Could you check a few things on this model? Use its own coordinates, in mm. A direction names the side the tool comes from. Round coordinates to 2 decimals unless told otherwise and drop trailing zeros. Write each loop counter-clockwise with the first axis right and the second up, starting at its lowest first coordinate (ties: lowest second). Pieces come first, ordered by that corner, then holes. Notation, with made-up numbers: M 14,60.5 L 52,60.5 A29 ccw 52,83.5 Z; hole C 46,-30.75 d11. An arc over 180 degrees is marked long. One line per item, written item: value. Start each with the question number.
(1) I want a section at A-A on y = -12. Please give me the cut outline in (x, z).
(2) Which directions (+Z, -Z, +X, -X, +Y, -Y) give clear straight access to the entire face, cutting with the end or side of a thin tool? Please do faces 1 (the face through (9.13, 17.26, -17.32)), 2 (the face through (75, -10, -68)), 3 (the face through (51, -10, -140)).
(3) Thinking about a two-plate mould opening in Y: for faces 4 (the face through (21, 75, -136)), 5 (the face through (29.84, 82.5, -120.4)), 6 (the face through (82.13, -9.86, -123.07)), which applies, released by +Y, released by -Y, zero draft, split by the parting line, or undercut?
(4) I'm going to push flat-ended pins straight in: pin 1 Ø12 at (x, y) = (23, 56) entering from -Z; pin 2 Ø7.5 at (x, z) = (6.5, -8) entering from +Y; pin 3 Ø16 at (x, y) = (49.5, -6.5) entering from -Z; pin 4 Ø13.5 at (x, z) = (85, -130) entering from -Y. Where does each tip first touch, or does it pass through?
(5) I want a section at D-D on x = 7.5. Please give me the cut outline in (y, z).
(6) I want a section at C-C on z = -125.5. Please give me the cut outline in (x, y), and give its area (3 significant figures).
(7) If I drill on L1, parallel to X at y = 3.5, z = -9.5; L2, parallel to X at y = -15.5, z = -130; L3, parallel to Z at x = 56, y = -9.5, over which ranges is the centre line in solid material (lowest first)?
(8) I want a section at B-B on x = 56. Please give me the cut outline in (y, z).
```python
from build123d import *

# Parameters (mm, degrees)
SKETCH1_R            = 7.5
BOSS_EXTRUDE9_DEPTH  = 20
SKETCH3_R            = 7.5
BOSS_EXTRUDE10_DEPTH = 35
SKETCH5_W            = 20
SKETCH5_H            = 20
BOSS_EXTRUDE11_DEPTH = 55
CUT_EXTRUDE2_DEPTH   = 228.774559598
BOSS_EXTRUDE13_START = 75
SKETCH10_R           = 10
BOSS_EXTRUDE13_DEPTH = 75
SKETCH12_W           = 25
SKETCH12_H           = 25
BOSS_EXTRUDE14_DEPTH = 15
SKETCH21_R           = 7.5
CUT_EXTRUDE8_DEPTH   = 8


with BuildPart() as part:
    # Sketch1 → Boss-Extrude9 (new body)
    with BuildSketch(Plane(origin=(0, 0, 0), x_dir=(1, 0, 0), z_dir=(0, 1, 0))):
        with BuildLine():
            Line((0, 0), (170, 0))
            Line((170, 0), (170, 20))
            Line((170, 20), (95, 20))
            Line((95, 20), (95, 115.638593384))
            ThreePointArc((95, 115.638593384), (85, 147.5), (75, 115.638593384))
            Line((75, 115.638593384), (75, 20))
            Line((75, 20), (0, 20))
            Line((0, 20), (0, 0))
        make_face()
        with Locations(Location((85, 130, 0), (0, 0, 270))):
            Circle(SKETCH1_R, mode=Mode.SUBTRACT)
    extrude(amount=-BOSS_EXTRUDE9_DEPTH)

    # Sketch3 → Boss-Extrude10 (add)
    with BuildSketch(Plane(origin=(0, 0, 0), x_dir=(1, 0, 0), z_dir=(0, 1, 0))):
        with Locations(Location((7.5, 10, 0), (0, 0, 180))):
            Circle(SKETCH3_R)
        with Locations((162.5, 10)):
            Circle(SKETCH3_R)
    extrude(amount=BOSS_EXTRUDE10_DEPTH)

    # Sketch5 → Boss-Extrude11 (add)
    with BuildSketch(Plane.ZY.offset(-75)):
        with Locations((-130, -10)):
            Rectangle(SKETCH5_W, SKETCH5_H)
    extrude(amount=BOSS_EXTRUDE11_DEPTH)

    # Sketch6 → Cut-Extrude2 (cut, through all)
    with BuildSketch(Plane(origin=(0, 0, 0), x_dir=(1, 0, 0), z_dir=(0, 1, 0))):
        with BuildLine():
            Line((20, 130), (20, 120))
            Line((20, 120), (30, 120))
            ThreePointArc((30, 120), (22.928932188, 122.928932188), (20, 130))
        make_face()
        with BuildLine():
            Line((20, 140), (20, 130))
            ThreePointArc((20, 130), (22.928932188, 137.071067812), (30, 140))
            Line((30, 140), (20, 140))
        make_face()
    extrude(amount=-CUT_EXTRUDE2_DEPTH, mode=Mode.SUBTRACT)

    # Sketch10 → Boss-Extrude13 (add)
    with BuildSketch(Plane(origin=(0, 0, 0), x_dir=(1, 0, 0), z_dir=(0, 1, 0)).offset(BOSS_EXTRUDE13_START)):
        with Locations(Location((30, 130, 0), (0, 0, 270))):
            Circle(SKETCH10_R)
    extrude(amount=-BOSS_EXTRUDE13_DEPTH)

    # Sketch12 → Boss-Extrude14 (add)
    with BuildSketch(Plane(origin=(0, 75, 0), x_dir=(1, 0, 0), z_dir=(0, 1, 0))):
        with Locations((30, 130)):
            Rectangle(SKETCH12_W, SKETCH12_H)
    extrude(amount=BOSS_EXTRUDE14_DEPTH)

    # Sketch20 → Cut-Revolve5 (revolve, cut)
    with BuildSketch(Plane(origin=(0, 90, 0), x_dir=(1, 0, 0), z_dir=(0, 1, 0))):
        with BuildLine():
            Line((30, 140), (30, 120))
            ThreePointArc((30, 120), (40, 130), (30, 140))
        make_face()
    revolve(axis=Axis((30, 90, -140), (0, 0, 1)), mode=Mode.SUBTRACT)

    # Sketch21 → Cut-Extrude8 (cut)
    with BuildSketch(Plane.XY.offset(-117.5)):
        with Locations((30, 90)):
            Circle(SKETCH21_R)
    extrude(amount=-CUT_EXTRUDE8_DEPTH, mode=Mode.SUBTRACT)


solid = part.part
```
Found:
1. outline: M 0,-20 L 75,-20 L 75,-115.64 A17.5 ccw 70.64,-120 L 30,-120 A10 ccw 30,-140 L 70.64,-140 A17.5 ccw long 95,-115.64 L 95,-20 L 170,-20 L 170,0 L 0,0 Z; hole C 85,-130 d15
2. face 1: +Y
2. face 2: -X, +Y, -Y
2. face 3: -Z, -X, -Y
3. face 4: undercut
3. face 5: released by +Y
3. face 6: zero draft
4. pin 1: stops at z = -139.95
4. pin 2: stops at y = 35
4. pin 3: stops at z = -140
4. pin 4: passes through
5. outline: M -20,-20 L 0,-20 L 0,-17.5 L 35,-17.5 L 35,-2.5 L 0,-2.5 L 0,0 L -20,0 Z
6. outline: M 17.5,75 L 21.07,75 L 21.07,-20 L 79,-20 L 79,0 L 38.93,0 L 38.93,75 L 42.5,75 L 42.5,90 L 38.93,90 A8.93 cw 21.07,90 L 17.5,90 Z; M 91,-20 L 101.91,-20 L 101.91,0 L 91,0 Z
6. area: 2,970 mm²
7. L1: x = 0.02 to 14.98, 155.02 to 169.98
7. L2: x = 20 to 77.5, 92.5 to 102.5
7. L3: z = -140 to -120, -20 to 0
8. outline: M -20,-140 L 0,-140 L 0,-120 L -20,-120 Z; M -20,-20 L 0,-20 L 0,0 L -20,0 Z
